from build123d import *

# Parameters (mm, degrees)
F0_W     = 152.4
F0_H     = 152.4
F1_DEPTH = 12.7
F2_W     = 50.8
F2_H     = 50.8
F3_DEPTH = 304.8
F4_W     = 38.1
F4_H     = 36.661644
F5_DEPTH = 304.8
F6_R     = 6.35
F7_W     = 15.875
F7_H     = 25.4
F8_DEPTH = 12.701


with BuildPart() as f1:
    # F0 (on Right) → F1 (new body)
    with BuildSketch(Plane.YZ):
        Rectangle(F0_W, F0_H)
    extrude(amount=-F1_DEPTH)

    # F2 (on face) → F3 (join)
    with BuildSketch(Plane.YZ):
        Rectangle(F2_W, F2_H)
    extrude(amount=F3_DEPTH)

    # F4 (on face) → F5 (cut, through all)
    with BuildSketch(Plane.YZ.offset(304.8)):
        Rectangle(F4_W, F4_H)
    extrude(amount=-F5_DEPTH, mode=Mode.SUBTRACT)

    # F6
    f6_edges = [f1.edges().sort_by_distance(p)[0] for p in [
        (152.4, -25.4, 25.4),
        (152.4, 25.4, 25.4),
        (152.4, -25.4, -25.4),
        (152.4, 25.4, -25.4),
    ]]
    fillet(f6_edges, radius=F6_R)

    # F7 (on face) → F8 (cut, through all)
    with BuildSketch(Plane.YZ):
        with Locations((-57.15, 50.8)):
            Rectangle(F7_W, F7_H)
        with Locations((57.15, 50.8)):
            Rectangle(F7_W, F7_H)
        with Locations((57.15, -50.8)):
            Rectangle(F7_W, F7_H)
        with Locations((-57.15, -50.8)):
            Rectangle(F7_W, F7_H)
    extrude(amount=-F8_DEPTH, mode=Mode.SUBTRACT)


solid = f1.part
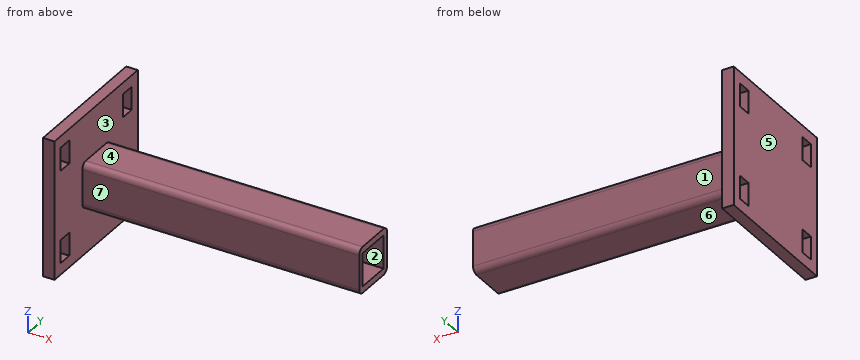
Here's how the part is built. I have some questions about the finished solid (model axes, mm). Face numbers are marked on the shaded views. A direction names the side the tool comes from. Round coordinates to 2 decimals unless told otherwise and drop trailing zeros. Write each loop counter-clockwise with the first axis right and the second up, starting at its lowest first coordinate (ties: lowest second). Pieces come first, ordered by that corner, then holes.
1. Will these pins go through, and if not, where does the flat tip stop? pin 1 Ø11.5 at (x, y) = (80, 9) entering from +Z; pin 2 Ø3 at (y, z) = (-51.5, -41.5) entering from -X; pin 3 Ø5 at (y, z) = (-19, 9) entering from +X; pin 4 Ø10 at (y, z) = (-47, 48) entering from +X.
2. Suppose I cut it at B-B (x = 104.5). List the corners of the cut face in (y, z) for me, and give its area (3 significant figures).
3. Suppose I cut it at A-A (z = 57.5). List the corners of the cut face in (x, y) for me.
4. Suppose I cut it at D-D (y = 1.5). List the corners of the cut face in (x, z) for me, and give its area (3 significant figures).
5. Suppose I cut it at C-C (z = 8). List the corners of the cut face in (x, y) for me.
6. For the marked faces 4, 5, 6 and 7, which set-ups out of +Z, -Z, +X, -X, +Y, -Y let a thin tool reach every point of the face, with its end or its side?
7. If we mould it in two halves opening along Y, with no side actions, what happens to the marked faces 1, 2 and 3? For each: released by +Y, released by -Y, zero draft, split by the parting line, or undercut.
8. I need wall thicknesses on L1, parallel to Y at x = 292, z = -1.5; L2, parallel to X at y = 21.5, z = -50; L3, parallel to Z at x = 225.5, y = -5. Which ranges of each line are inside material? Lowest first, please.
Answer sheet:
1. pin 1: stops at z = 25.4
1. pin 2: passes through
1. pin 3: stops at x = 304.8
1. pin 4: stops at x = 0
2. outline: (-25.4, -19.05) arc R6.35 ccw to (-19.05, -25.4) - (19.05, -25.4) arc R6.35 ccw to (25.4, -19.05) - (25.4, 19.05) arc R6.35 ccw to (19.05, 25.4) - (-19.05, 25.4) arc R6.35 ccw to (-25.4, 19.05) - close; hole (-19.05, -18.33) - (19.05, -18.33) - (19.05, 18.33) - (-19.05, 18.33) - close
2. area: 1,150 mm2
3. outline: (-12.7, -76.2) - (0, -76.2) - (0, -65.09) - (-12.7, -65.09) - close; (-12.7, -49.21) - (0, -49.21) - (0, 49.21) - (-12.7, 49.21) - close; (-12.7, 65.09) - (0, 65.09) - (0, 76.2) - (-12.7, 76.2) - close
4. outline: (-12.7, -76.2) - (0, -76.2) - (0, -25.4) - (304.8, -25.4) - (304.8, -18.33) - (0, -18.33) - (0, 18.33) - (304.8, 18.33) - (304.8, 25.4) - (0, 25.4) - (0, 76.2) - (-12.7, 76.2) - close
4. area: 6,240 mm2
5. outline: (-12.7, -76.2) - (0, -76.2) - (0, -25.4) - (304.8, -25.4) - (304.8, -19.05) - (0, -19.05) - (0, 19.05) - (304.8, 19.05) - (304.8, 25.4) - (0, 25.4) - (0, 76.2) - (-12.7, 76.2) - close
6. face 4: +Z, +X, +Y, -Y
6. face 5: +Z, -Z, -X, +Y, -Y
6. face 6: -Z, +X, +Y, -Y
6. face 7: +Z, -Z, +X, -Y
7. face 1: released by +Y
7. face 2: undercut
7. face 3: zero draft
8. L1: y = -25.4 to -19.05, 19.05 to 25.4
8. L2: x = -12.7 to 0
8. L3: z = -25.4 to -18.33, 18.33 to 25.4
